Could you check a few things on this model? Use its own coordinates, in mm. Give positions to 0.01 mm unless a question says otherwise; leave off trailing zeros. Order: outer loops, then holes, each group sorted by start corner. A loop starts at its lowest first (then second) coordinate and runs counter-clockwise, first axis right, second up. Notation, with made-up numbers: (47.5, 54.5) - (78.5, 54.5) arc R25 cw to (78.5, 74.5) - close; hole circle Ø5 at (47.5, 87). An arc over 180 degrees is marked (long way). One line per question, with ' | ' between items. Start each with the question number.
1. Imagine slicing it at A-A (z = 2.35). Give the number of separate pieces and of enclosed holes in the cut face, and give its area (3 significant figures).
2. Imagine slicing it at B-B (y = -5). Please give me the cut outline in (x, z).
3. I need wall thicknesses on probe 1 along X at (y, z) = (5.25, 4.45); probe 2 along X at (y, z) = (3, 2.4); probe 3 along Y at (x, z) = (4.5, 2.1). Which ranges of each line are inside material? Lowest first, please. Write a range as from..to.
4. For P1, Ø3, axis at x = -3.3, y = -4.1, coming from the +Z side, with a flat end and sliding along its axis, tell me the tip position at first contact or that it passes through.
```python
from build123d import *

# Parameters (mm, degrees)
F1_DEPTH = 4.7625


# Not quite as in the source:
# - a length typed as a fraction of an inch, garbled in the dataset ("3 / 203.2 mm" for 3/8 in), is restored


with BuildPart() as f1:
    # F0 (on Top) → F1 (new body)
    with BuildSketch(Plane.XY):
        with BuildLine():
            Line((-3.302, 5.9590800321), (-3.302, 7.747))
            Line((-3.302, 7.747), (-29.464, 7.747))
            Line((-29.464, 7.747), (-29.464, 5.9590800321))
            ThreePointArc((-29.464, 5.9590800321), (-28.2067641431, 5.4383158891), (-27.686, 4.1810800321))
            ThreePointArc((-27.686, 4.1810800321), (-28.2067641431, 2.9238441752), (-29.464, 2.4030800321))
            Line((-29.464, 2.4030800321), (-29.464, -2.3199413316))
            ThreePointArc((-29.464, -2.3199413316), (-28.2067641431, -2.8407054746), (-27.686, -4.0979413316))
            ThreePointArc((-27.686, -4.0979413316), (-28.2067641431, -5.3551771885), (-29.464, -5.8759413316))
            Line((-29.464, -5.8759413316), (-29.464, -7.747))
            Line((-29.464, -7.747), (-3.302, -7.747))
            Line((-3.302, -7.747), (-3.302, -5.8759413316))
            ThreePointArc((-3.302, -5.8759413316), (-5.08, -4.0979413316), (-3.302, -2.3199413316))
            Line((-3.302, -2.3199413316), (-3.302, 2.4030800321))
            ThreePointArc((-3.302, 2.4030800321), (-5.08, 4.1810800321), (-3.302, 5.9590800321))
        make_face()
        with BuildLine():
            Line((-29.464, 5.9590800321), (-29.464, 7.747))
            Line((-29.464, 7.747), (-33.02, 7.747))
            Line((-33.02, 7.747), (-33.02, -7.747))
            Line((-33.02, -7.747), (-29.464, -7.747))
            Line((-29.464, -7.747), (-29.464, -5.8759413316))
            ThreePointArc((-29.464, -5.8759413316), (-31.242, -4.0979413316), (-29.464, -2.3199413316))
            Line((-29.464, -2.3199413316), (-29.464, 2.4030800321))
            ThreePointArc((-29.464, 2.4030800321), (-31.242, 4.1810800321), (-29.464, 5.9590800321))
        make_face()
        with BuildLine():
            Line((29.464, 5.9590800321), (29.464, 7.747))
            Line((29.464, 7.747), (3.302, 7.747))
            Line((3.302, 7.747), (3.302, 5.9590800321))
            ThreePointArc((3.302, 5.9590800321), (4.5592358569, 5.4383158891), (5.08, 4.1810800321))
            ThreePointArc((5.08, 4.1810800321), (4.5592358569, 2.9238441752), (3.302, 2.4030800321))
            Line((3.302, 2.4030800321), (3.302, -2.3199413316))
            ThreePointArc((3.302, -2.3199413316), (4.5592358569, -2.8407054746), (5.08, -4.0979413316))
            ThreePointArc((5.08, -4.0979413316), (4.5592358569, -5.3551771885), (3.302, -5.8759413316))
            Line((3.302, -5.8759413316), (3.302, -7.747))
            Line((3.302, -7.747), (29.464, -7.747))
            Line((29.464, -7.747), (29.464, -5.8759413316))
            ThreePointArc((29.464, -5.8759413316), (27.686, -4.0979413316), (29.464, -2.3199413316))
            Line((29.464, -2.3199413316), (29.464, 2.4030800321))
            ThreePointArc((29.464, 2.4030800321), (27.686, 4.1810800321), (29.464, 5.9590800321))
        make_face()
        with BuildLine():
            Line((33.02, -7.747), (33.02, 7.747))
            Line((33.02, 7.747), (29.464, 7.747))
            Line((29.464, 7.747), (29.464, 5.9590800321))
            ThreePointArc((29.464, 5.9590800321), (30.7212358569, 5.4383158891), (31.242, 4.1810800321))
            ThreePointArc((31.242, 4.1810800321), (30.7212358569, 2.9238441752), (29.464, 2.4030800321))
            Line((29.464, 2.4030800321), (29.464, -2.3199413316))
            ThreePointArc((29.464, -2.3199413316), (30.7212358569, -2.8407054746), (31.242, -4.0979413316))
            ThreePointArc((31.242, -4.0979413316), (30.7212358569, -5.3551771885), (29.464, -5.8759413316))
            Line((29.464, -5.8759413316), (29.464, -7.747))
            Line((29.464, -7.747), (33.02, -7.747))
        make_face()
        with BuildLine():
            Line((3.302, 5.9590800321), (3.302, 7.747))
            Line((3.302, 7.747), (-3.302, 7.747))
            Line((-3.302, 7.747), (-3.302, 5.9590800321))
            ThreePointArc((-3.302, 5.9590800321), (-2.0447641431, 5.4383158891), (-1.524, 4.1810800321))
            ThreePointArc((-1.524, 4.1810800321), (-2.0447641431, 2.9238441752), (-3.302, 2.4030800321))
            Line((-3.302, 2.4030800321), (-3.302, -2.3199413316))
            ThreePointArc((-3.302, -2.3199413316), (-2.0447641431, -2.8407054746), (-1.524, -4.0979413316))
            ThreePointArc((-1.524, -4.0979413316), (-2.0447641431, -5.3551771885), (-3.302, -5.8759413316))
            Line((-3.302, -5.8759413316), (-3.302, -7.747))
            Line((-3.302, -7.747), (3.302, -7.747))
            Line((3.302, -7.747), (3.302, -5.8759413316))
            ThreePointArc((3.302, -5.8759413316), (1.524, -4.0979413316), (3.302, -2.3199413316))
            Line((3.302, -2.3199413316), (3.302, 2.4030800321))
            ThreePointArc((3.302, 2.4030800321), (1.524, 4.1810800321), (3.302, 5.9590800321))
        make_face()
    extrude(amount=F1_DEPTH)


solid = f1.part
```
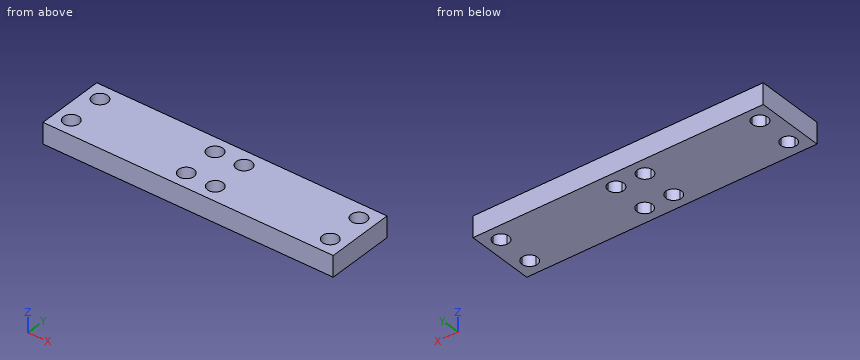
Results found:
1) separate pieces: 1 | enclosed holes: 8 | area: 944 mm2
2) outline: (-33.02, 0) - (-31, 0) - (-31, 4.76) - (-33.02, 4.76) - close; (-27.93, 0) - (-4.83, 0) - (-4.83, 4.76) - (-27.93, 4.76) - close; (-1.77, 0) - (1.77, 0) - (1.77, 4.76) - (-1.77, 4.76) - close; (4.83, 0) - (27.93, 0) - (27.93, 4.76) - (4.83, 4.76) - close; (31, 0) - (33.02, 0) - (33.02, 4.76) - (31, 4.76) - close
3) probe 1: x = -33.02..-30.88, -28.04..-4.72, -1.88..1.88, 4.72..28.04, 30.88..33.02 | probe 2: x = -33.02..-30.79, -28.13..-4.63, -1.97..1.97, 4.63..28.13, 30.79..33.02 | probe 3: y = -7.75..-5.41, -2.78..2.87, 5.49..7.75
4) P1: passes through
